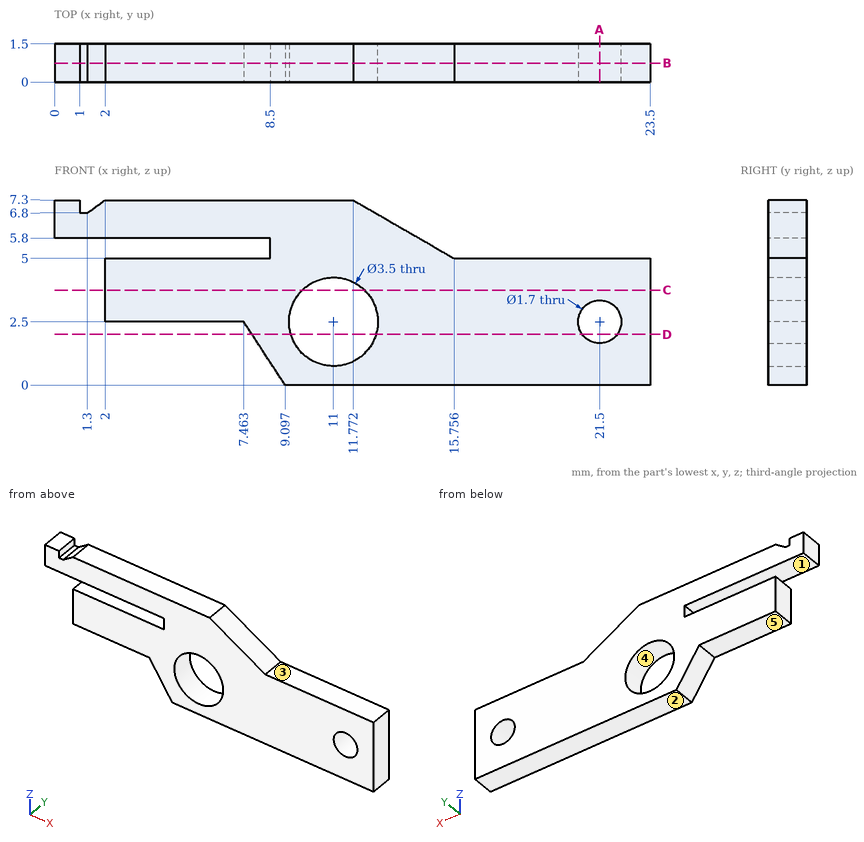
For this review, use the dimensioned drawing (mm, ordinates from the lowest corner) and the shaded views. A direction names the side the tool comes from. Round coordinates to 2 decimals unless told otherwise and drop trailing zeros. Order: outer loops, then holes, each group sorted by start corner. A loop starts at its lowest first (then second) coordinate and runs counter-clockwise, first axis right, second up. Notation, with made-up numbers: (-27, 65) -> (20, 65) arc R7 cw to (20, 72) -> close; hole circle Ø7 at (54.25, 82.25). An arc over 180 degrees is marked (long way). Use CSV: the item, a comma, the result in double quotes. Start each with the question number.
(1) Consider section C-C on z = 3.75. Write out the cut boundary in (x, y) (1 decimal).
(2) Wall thickness on probe 1 along Z at (x, y) = (11, 0.7); probe 2 along Z at (x, y) = (21.5, 1.1); probe 3 along Z at (x, y) = (19.75, 1.15): over which ranges is each line inside the solid? List them lowest first. Write a range as from..to.
(3) Consider section A-A on x = 21.5. Write out the cut boundary in (y, z).
(4) Consider section B-B on y = 0.75. State how many separate pieces and enclosed holes the cut face has.
(5) Tool access review of the marked faces 1 and 2: name each direction out of +Z, -Z, +X, -X, +Y, -Y from which nothing blocks a thin tool from reaching the whole face with its end or side.
(6) Mouldability with a two-part tool opening along Z and no side actions: class the marked faces 3, 4 and 5 as pulls with the +Z half, pulls with the -Z half, needs draft (parallel to the pull), parting line crosses it, or undercut.
(7) Insertion check: pin 1 (4 mm diameter, centred on x = 11, z = 2.5, fed in from +Y). The pin has a flat end and moves straight along its axis. Give the tip position at first contact, or say it passes through.
(8) Consider section D-D on z = 2. Write out the cut boundary in (x, y).
Responses:
1,outline,"(2, 0) -> (9.8, 0) -> (9.8, 1.5) -> (2, 1.5) -> close; (12.2, 0) -> (23.5, 0) -> (23.5, 1.5) -> (12.2, 1.5) -> close"
2,probe 1,"0..0.75, 4.25..7.3"
2,probe 2,"0..1.65, 3.35..5"
2,probe 3,"0..5"
3,outline,"(0, 0) -> (1.5, 0) -> (1.5, 1.65) -> (0, 1.65) -> close; (0, 3.35) -> (1.5, 3.35) -> (1.5, 5) -> (0, 5) -> close"
4,separate pieces,"1"
4,enclosed holes,"2"
5,face 1,"-X, +Y, -Y"
5,face 2,"-Z, +X, -X, +Y, -Y"
6,face 3,"pulls with the +Z half"
6,face 4,"undercut"
6,face 5,"pulls with the -Z half"
7,pin 1,"y = 1.5"
8,outline,"(7.79, 0) -> (9.32, 0) -> (9.32, 1.5) -> (7.79, 1.5) -> close; (12.68, 0) -> (20.81, 0) -> (20.81, 1.5) -> (12.68, 1.5) -> close; (22.19, 0) -> (23.5, 0) -> (23.5, 1.5) -> (22.19, 1.5) -> close"
